Verification items for the finished model (mm, model axes). Face numbers are marked on the shaded views. A direction names the side the tool comes from. Round coordinates to 2 decimals unless told otherwise and drop trailing zeros. Loops run counter-clockwise (first coordinate to the right, second up) from the corner with the lowest first, then second, coordinate; pieces in that order, holes last. Notation, with made-up numbers: (70, -35.75) - (99, -35.75) arc R24 ccw to (99, -12.75) - close; hole circle Ø7 at (-34.5, -30.5). An arc over 180 degrees is marked (long way). Use a Markdown table: item, result. Add a question column.
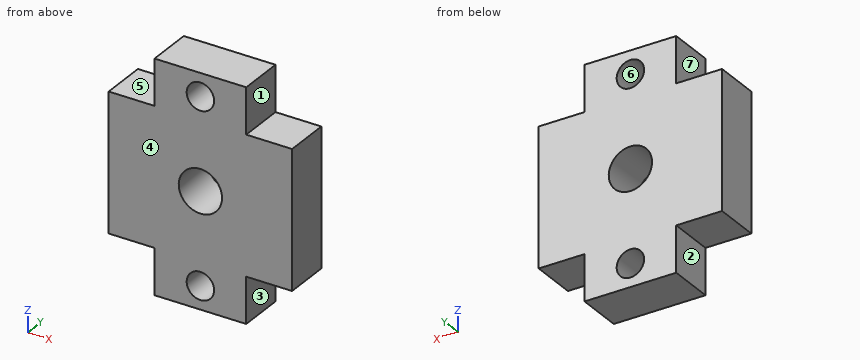
```python
from build123d import *

# Parameters (mm, degrees)
SKETCH1_W               = 25.4
SKETCH1_H               = 31.75
BOSS_EXTRUDE1_DEPTH     = 3.175
CUT_EXTRUDE1_REACH      = 23.299
SKETCH2_W               = 6.35
SKETCH2_H               = 6.35
MIRROR2_COPY_1_REACH    = 23.299
MIRROR2_COPY_1_SKETCH_W = 6.35
MIRROR2_COPY_1_SKETCH_H = 6.35
CUT_EXTRUDE2_REACH      = 23.299
SKETCH5_R               = 3


with BuildPart() as part:
    # Sketch1 → Boss-Extrude1 (new, symmetric)
    with BuildSketch(Plane(origin=(0, 0, 0), x_dir=(1, 0, 0), z_dir=(0, 1, 0))):
        Rectangle(SKETCH1_W, SKETCH1_H)
    extrude(amount=BOSS_EXTRUDE1_DEPTH, both=True)

    # Sketch2 → Cut-Extrude1 (cut, up to next)
    with BuildSketch(Plane(origin=(0, 3.175, 0), x_dir=(1, 0, 0), z_dir=(0, 1, 0)), mode=Mode.PRIVATE) as cut_extrude1_sk1:
        with Locations((-9.525, 12.7)):
            Rectangle(SKETCH2_W, SKETCH2_H)
    cut_extrude1_tool1 = extrude(cut_extrude1_sk1.sketch, amount=-CUT_EXTRUDE1_REACH, mode=Mode.PRIVATE) & part.part
    cut_extrude1 = cut_extrude1_tool1.solids().sort_by_distance((-9.525, 3.175, -12.7))[0]
    add(cut_extrude1, mode=Mode.SUBTRACT)

    # Mirror1: Cut-Extrude1 across plane
    add(cut_extrude1.mirror(Plane.XY), mode=Mode.SUBTRACT)

    # Mirror2: Cut-Extrude1 across plane
    add(cut_extrude1.mirror(Plane(origin=(0, 0, 0), x_dir=(0, 0, 1), z_dir=(1, 0, 0))), mode=Mode.SUBTRACT)

    # Mirror2 copy 1 sketch → Mirror2 copy 1 (cut, up to next)
    with BuildSketch(Plane(origin=(0, 3.175, 0), x_dir=(-1, 0, 0), z_dir=(0, 1, 0)), mode=Mode.PRIVATE) as mirror2_copy_1_sk1:
        with Locations((-9.525, 12.7)):
            Rectangle(MIRROR2_COPY_1_SKETCH_W, MIRROR2_COPY_1_SKETCH_H)
    mirror2_copy_1_tool1 = extrude(mirror2_copy_1_sk1.sketch, amount=-MIRROR2_COPY_1_REACH, mode=Mode.PRIVATE) & part.part
    add(mirror2_copy_1_tool1.solids().sort_by_distance((9.525, 3.175, 12.7))[0], mode=Mode.SUBTRACT)

    # Sketch3 → #6 Clearance Hole1 (revolve, cut)
    with BuildSketch(Plane(origin=(0, 3.175, -12.7), x_dir=(0, 0, 1), z_dir=(1, 0, 0))):
        Polygon((0, 0), (0, 7.490824014), (1.89865, 6.35), (1.89865, 0), align=None)
    f_6_clearance_hole1 = revolve(axis=Axis((0, 9.525, -12.7), (0, -1, 0)), mode=Mode.SUBTRACT)

    # Mirror3: #6 Clearance Hole1 across plane
    add(f_6_clearance_hole1.mirror(Plane.XY), mode=Mode.SUBTRACT)

    # Sketch5 → Cut-Extrude2 (cut, up to next)
    with BuildSketch(Plane(origin=(0, 3.175, 0), x_dir=(1, 0, 0), z_dir=(0, 1, 0)), mode=Mode.PRIVATE) as cut_extrude2_sk1:
        with Locations(Location((0, 0, 0), (0, 0, 270))):
            Circle(SKETCH5_R)
    cut_extrude2_tool1 = extrude(cut_extrude2_sk1.sketch, amount=-CUT_EXTRUDE2_REACH, mode=Mode.PRIVATE) & part.part
    add(cut_extrude2_tool1.solids().sort_by_distance((0, 3.175, 0))[0], mode=Mode.SUBTRACT)


solid = part.part
```
Q1. Section check A-A on x = 0. Record the cut outline in (y, z) (3 decimals), plus the area to 3 significant figures.
Q2. Section check D-D on z = 0. Record the cut outline in (x, y) (3 decimals).
Q3. Go/stop test with flat-tipped pins: pin 1 Ø3 at (y, z) = (-0.5, -11.5) entering from -X; pin 2 Ø10 at (x, z) = (-0.5, -0.5) entering from +Y (3 decimals); pin 3 Ø1.9 at (x, y) = (8.5, -1) entering from +Z (3 decimals); pin 4 Ø2.5 at (x, z) = (0, 12.7) entering from +Y. Record where each tip stops, or that it passes through.
Q4. Set-up check for the marked faces 1, 2, 3 and 4: record each of +Z, -Z, +X, -X, +Y, -Y from which the full face is reachable in a straight line by a thin tool's end or side.
Q5. Section check C-C on y = 1.25. Record the cut outline in (x, z) (3 decimals).
Q6. Release check for a two-part mould opening along Z. For the marked faces 5, 6 and 7 record: +Z half, -Z half, draft (parallel to the pull), parting line (faces both ways), or undercut.
Q7. Thickness scan on line 1 along X through (y, z) = (0.5, -12.7); line 2 along X through (y, z) = (1, 0); line 3 along Z through (x, y) = (9.5, -0.5) (3 decimals). Record the ranges inside material, lowest first.
Q8. Section check B-B on z = 12.7. Record the cut outline in (x, y) (3 decimals).
Determined:
| question | item | result |
|---|---|---|
| 1 | outline | (-3.175, -15.875) - (3.175, -15.875) - (3.175, -14.599) - (-3.175, -14.599) - close; (-3.175, -10.801) - (3.175, -10.801) - (3.175, -3) - (-3.175, -3) - close; (-3.175, 3) - (3.175, 3) - (3.175, 10.801) - (-3.175, 10.801) - close; (-3.175, 14.599) - (3.175, 14.599) - (3.175, 15.875) - (-3.175, 15.875) - close |
| 1 | area | 115 mm² |
| 2 | outline | (-12.7, -3.175) - (-3, -3.175) - (-3, 3.175) - (-12.7, 3.175) - close; (3, -3.175) - (12.7, -3.175) - (12.7, 3.175) - (3, 3.175) - close |
| 3 | pin 1 | stops at x = -6.35 |
| 3 | pin 2 | stops at y = 3.175 |
| 3 | pin 3 | stops at z = 9.525 |
| 3 | pin 4 | passes through |
| 4 | face 1 | +Z, +X, +Y, -Y |
| 4 | face 2 | -Z, -X, +Y, -Y |
| 4 | face 3 | -Z, +X, +Y, -Y |
| 4 | face 4 | +Z, -Z, +X, -X, -Y |
| 5 | outline | (-12.7, -9.525) - (-6.35, -9.525) - (-6.35, -15.875) - (6.35, -15.875) - (6.35, -9.525) - (12.7, -9.525) - (12.7, 9.525) - (6.35, 9.525) - (6.35, 15.875) - (-6.35, 15.875) - (-6.35, 9.525) - (-12.7, 9.525) - close; hole circle Ø6 at (0, 0); hole circle Ø3.797 at (0, -12.7); hole circle Ø3.797 at (0, 12.7) |
| 6 | face 5 | +Z half |
| 6 | face 6 | undercut |
| 6 | face 7 | draft |
| 7 | line 1 | x = -6.35 to -1.9, 1.9 to 6.35 |
| 7 | line 2 | x = -12.7 to -3, 3 to 12.7 |
| 7 | line 3 | z = -9.525 to 9.525 |
| 8 | outline | (-6.35, -3.175) - (-1.899, -3.175) - (-1.899, 3.175) - (-6.35, 3.175) - close; (1.899, -3.175) - (6.35, -3.175) - (6.35, 3.175) - (1.899, 3.175) - close |
